CAD build for the part. Positions are in the model's coordinates, mm. A direction names the side the tool comes from. Give positions to 0.01 mm unless a question says otherwise; leave off trailing zeros. Loops run counter-clockwise (first coordinate to the right, second up) from the corner with the lowest first, then second, coordinate; pieces in that order, holes last.
```python
from build123d import *

# Parameters (mm, degrees)
SKETCH1_W           = 19.8
SKETCH1_H           = 15
SKETCH1_R           = 1.15
BOSS_EXTRUDE1_DEPTH = 3
SKETCH2_W           = 19.8
SKETCH2_H           = 3
BOSS_EXTRUDE2_DEPTH = 26
CHAMFER1_SIZE       = 3
CUT_EXTRUDE1_DEPTH  = 15
CHAMFER2_SIZE       = 4


with BuildPart() as part:
    # Sketch1 → Boss-Extrude1 (new body)
    with BuildSketch(Plane.XY):
        with Locations((0, 6.287671233)):
            Rectangle(SKETCH1_W, SKETCH1_H)
        with Locations((-4.75, 10.787671233)):
            Circle(SKETCH1_R, mode=Mode.SUBTRACT)
        with Locations(Location((4.75, 10.787671233, 0), (0, 0, 180))):
            Circle(SKETCH1_R, mode=Mode.SUBTRACT)
    extrude(amount=BOSS_EXTRUDE1_DEPTH)

    # Sketch2 → Boss-Extrude2 (add)
    with BuildSketch(Plane.XY.offset(3)):
        with Locations((0, 0.287671233)):
            Rectangle(SKETCH2_W, SKETCH2_H)
    extrude(amount=BOSS_EXTRUDE2_DEPTH)

    # Chamfer1
    chamfer1_edges = [part.edges().sort_by_distance(p)[0] for p in [
        (0, 1.787671233, 3),
        (-9.9, 13.787671233, 1.5),
        (9.9, 13.787671233, 1.5),
    ]]
    chamfer(chamfer1_edges, length=CHAMFER1_SIZE)

    # Sketch4 → Cut-Extrude1 (cut)
    with BuildSketch(Plane(origin=(0, 1.787671233, 0), x_dir=(1, 0, 0), z_dir=(0, 1, 0))):
        with BuildLine():
            Line((2.647058824, -22.5), (2.647058824, -9.5))
            ThreePointArc((2.647058824, -9.5), (4.797058824, -7.35), (6.947058824, -9.5))
            Line((6.947058824, -9.5), (6.947058824, -22.5))
            ThreePointArc((6.947058824, -22.5), (4.797058824, -24.65), (2.647058824, -22.5))
        make_face()
        with BuildLine():
            Line((-2.647058824, -22.5), (-2.647058824, -9.5))
            ThreePointArc((-2.647058824, -9.5), (-4.797058824, -7.35), (-6.947058824, -9.5))
            Line((-6.947058824, -9.5), (-6.947058824, -22.5))
            ThreePointArc((-6.947058824, -22.5), (-4.797058824, -24.65), (-2.647058824, -22.5))
        make_face()
    extrude(amount=-CUT_EXTRUDE1_DEPTH, mode=Mode.SUBTRACT)

    # Chamfer2
    chamfer2_edges = [part.edges().sort_by_distance(p)[0] for p in [
        (-9.9, 0.287671233, 29),
        (9.9, 0.287671233, 29),
    ]]
    chamfer(chamfer2_edges, length=CHAMFER2_SIZE)


solid = part.part
```
1. Probe line 1 along X through (y, z) = (-0.5, 13.5); line 2 along Y through (x, z) = (4.75, 0.7); line 3 along X through (y, z) = (1, 8). List the from-to ranges inside material, lowest first.
Responses:
line 1: x = -9.9 to -6.95, -2.65 to 2.65, 6.95 to 9.9
line 2: y = -1.21 to 9.64, 11.94 to 13.79
line 3: x = -9.9 to -6.34, -3.26 to 3.26, 6.34 to 9.9
2. Saw through at C-C, the plane y = 1.25. List the corners of the cut face in (x, z).
Responses:
outline: (-9.9, 0) - (9.9, 0) - (9.9, 25) - (5.9, 29) - (-5.9, 29) - (-9.9, 25) - close; hole (-6.95, 9.5) arc R2.15 ccw to (-2.65, 9.5) - (-2.65, 22.5) arc R2.15 ccw to (-6.95, 22.5) - close; hole (2.65, 9.5) arc R2.15 ccw to (6.95, 9.5) - (6.95, 22.5) arc R2.15 ccw to (2.65, 22.5) - close
3. Tool access for faces 4 (the face through (0, 1.788, 17)), 5 (the face through (5.66, 11.49, 1.48)), 6 (the face through (2.647, 0, 16)): list every direction of +Z, -Z, +X, -X, +Y, -Y with a clear straight run to the whole face (end or side of a thin tool).
Responses:
face 4: +Z, +X, -X, +Y
face 5: +Z, -Z
face 6: +Y, -Y
4. Saw through at D-D, the plane x = -2.25. List the corners of the cut face in (y, z), and give its area (4 significant figures).
Responses:
outline: (-1.21, 0) - (13.79, 0) - (13.79, 3) - (4.79, 3) - (1.79, 6) - (1.79, 29) - (-1.21, 29) - close
area: 127.5 mm2
5. Saw through at B-B, the plane z = 23. List the corners of the cut face in (x, y).
Responses:
outline: (-9.9, -1.21) - (-6.89, -1.21) - (-6.89, 1.79) - (-9.9, 1.79) - close; (-2.71, -1.21) - (2.71, -1.21) - (2.71, 1.79) - (-2.71, 1.79) - close; (6.89, -1.21) - (9.9, -1.21) - (9.9, 1.79) - (6.89, 1.79) - close
6. Pull direction X, two halves, no side cores. Call faces 1 (the face through (-2.647, 0, 16)), 2 (the face through (0, 0, 29)), 3 (the face through (-7.9, 0.3, 27)): released by +X, released by -X, zero draft, split by the parting line, or undercut.
Responses:
face 1: undercut
face 2: zero draft
face 3: released by -X
7. Saw through at A-A, the plane x = 4.75. List the corners of the cut face in (y, z), and give its area (3 significant figures).
Responses:
outline: (-1.21, 0) - (9.64, 0) - (9.64, 3) - (4.79, 3) - (1.79, 6) - (1.79, 7.35) - (-1.21, 7.35) - close; (-1.21, 24.65) - (1.79, 24.65) - (1.79, 29) - (-1.21, 29) - close; (11.94, 0) - (13.79, 0) - (13.79, 3) - (11.94, 3) - close
area: 68.7 mm2
8. Drop flat-ended pins along their axis: pin 1 (1.5 mm diameter, centred on x = 6, y = 10, fed in from +Z); pin 2 (5 mm diameter, centred on x = -5, z = 7, fed in from +Y); pin 3 (6 mm diameter, centred on x = -3.5, z = 21.5, fed in from +Y); pin 4 (2 mm diameter, centred on x = 4.75, y = 10.79, fed in from -Z). Give the stop position or say it passes through.
Responses:
pin 1: stops at z = 3
pin 2: stops at y = 3.29
pin 3: stops at y = 1.79
pin 4: passes through
